Could you check a few things on this drawing? It's one solid part, dimensions in mm from its lowest x, y, z. Coordinates: 2 decimals unless noted, no trailing zeros. Write each loop counter-clockwise with the first axis right and the second up, starting at its lowest first coordinate (ties: lowest second). Pieces come first, ordered by that corner, then holes.
Item 1: I want a section at C-C (x = 30). Please give me the cut outline in (y, z).
Item 2: I'm going to push flat-ended pins straight in: P1, Ø2.5, axis at x = 45.5, y = 6, coming from the +Z side; P2, Ø2.5, axis at y = 4.5, z = 2, coming from the -X side; P3, Ø4, axis at x = 6, y = 4, coming from the -Z side. Where does each tip first touch, or does it pass through?
Item 3: I want a section at D-D (y = 2.75). Please give me the cut outline in (x, z), and give its area (3 significant figures).
Item 4: If we mould it in two halves opening along Z, with no side actions, what happens to the marked faces 1 and 2? For each: pulls with the +Z half, pulls with the -Z half, needs draft (parallel to the pull), parting line crosses it, or undercut.
Item 5: I want a section at B-B (z = 50). Please give me the cut outline in (x, y).
Item 6: I want a section at A-A (y = 7). Please give me the cut outline in (x, z), and give its area (3 significant figures).
Item 7: Please list where these lines run through material, in increasing order: line 1 (Z direction, x = 30, y = 6); line 2 (Z direction, x = 37.5, y = 5.5); line 3 (X direction, y = 3.5, z = 39.5).
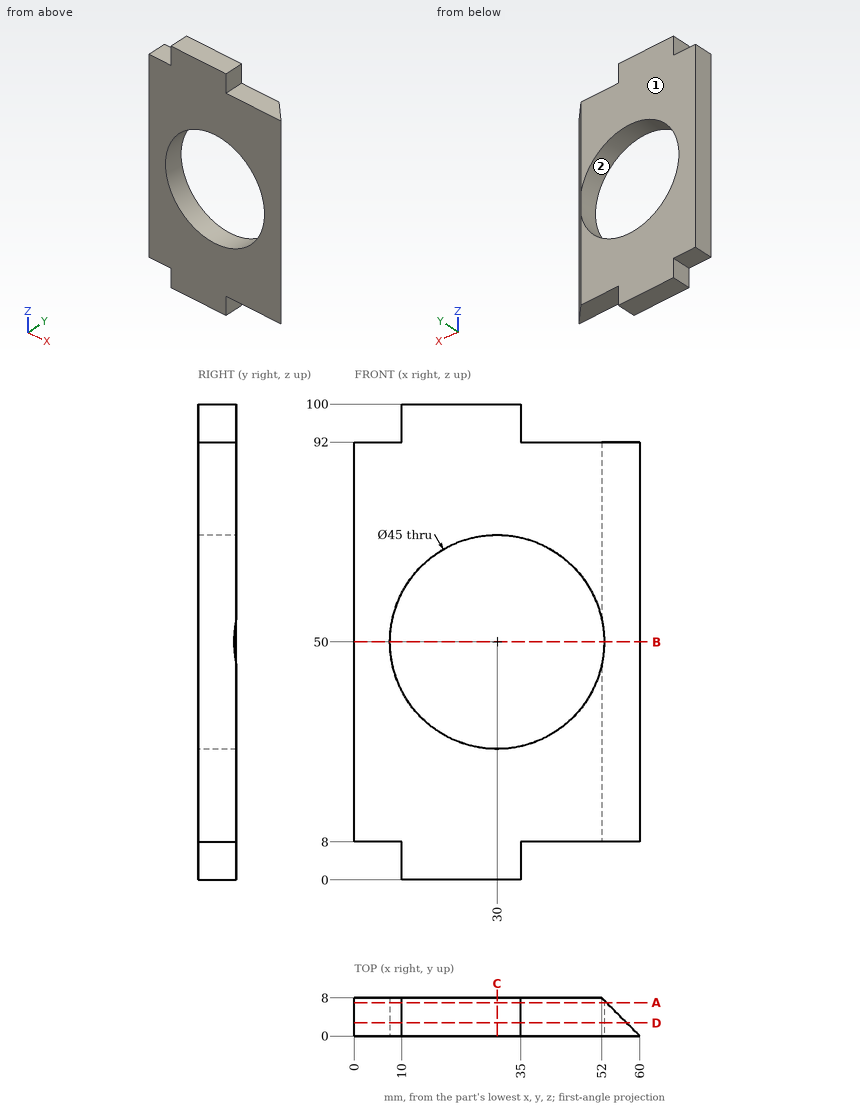
Answer:
1. outline: (0, 0) - (8, 0) - (8, 27.5) - (0, 27.5) - close; (0, 72.5) - (8, 72.5) - (8, 100) - (0, 100) - close
2. P1: stops at z = 92
2. P2: stops at x = 10
2. P3: stops at z = 8
3. outline: (0, 8) - (10, 8) - (10, 0) - (35, 0) - (35, 8) - (57.25, 8) - (57.25, 92) - (35, 92) - (35, 100) - (10, 100) - (10, 92) - (0, 92) - close; hole circle Ø45 at (30, 50)
3. area: 3,620 mm2
4. face 1: needs draft
4. face 2: undercut
5. outline: (0, 0) - (7.5, 0) - (7.5, 8) - (0, 8) - close; (52.5, 0) - (60, 0) - (52.5, 7.5) - close
6. outline: (0, 8) - (10, 8) - (10, 0) - (35, 0) - (35, 8) - (53, 8) - (53, 92) - (35, 92) - (35, 100) - (10, 100) - (10, 92) - (0, 92) - close; hole circle Ø45 at (30, 50)
6. area: 3,260 mm2
7. line 1: z = 0 to 27.5, 72.5 to 100
7. line 2: z = 8 to 28.79, 71.21 to 92
7. line 3: x = 0 to 10.1, 49.9 to 56.5
